Geometry check sheet. Reference: the model listing, model coordinates, mm. A direction names the side the tool comes from. Round coordinates to 2 decimals unless told otherwise and drop trailing zeros. Loops run counter-clockwise (first coordinate to the right, second up) from the corner with the lowest first, then second, coordinate; pieces in that order, holes last. Notation, with made-up numbers: (88, 36.25) - (130, 36.25) arc R24 cw to (130, 51.25) - close; hole circle Ø3 at (-32.5, 42). An arc over 180 degrees is marked (long way). Answer as CSV lines item,"result". Start each with the question number.
1) Thickness scan on line 1 along Y through (x, z) = (-45.25, 9.25); line 2 along X through (y, z) = (3.8, 14); line 3 along X through (y, z) = (0.25, 12.75). Record the ranges inside material, lowest first.
2) Access from +Z, -Z, +X, -X, +Y, -Y to the whole of each face (thin tool, end or side, straight path). Record for faces 1 (the flat face through (-49, 3, 13.787)), 2 (the flat face through (-48.043, 3, 8)), 3 (the flat face through (-50.143, 3, 8)), 4 (the cylindrical face through (-54.17, 1.49, 15.39)), 5 (the conical face through (-53.956, 0.191, 15.167)).
3) Cross-section at D-D on y = 1. Record the boundary of the cut face in (x, z), and give its area (3 significant figures).
4) Cross-section at C-C on z = 12. Record the boundary of the cut face in (x, y), and give its area (4 significant figures).
5) Depth check by flat-ended pin: P1, Ø1, axis at y = 3.5, z = 15, coming from the -X side; P2, Ø1.6, axis at y = 3, z = 8.5, coming from the +X side; P3, Ø1.6, axis at y = 4, z = 14.5, coming from the +X side. Enter the tip coordinate at first touch or a pass-through.
6) Cross-section at B-B on x = -52.75. Record the boundary of the cut face in (y, z).
7) Cross-section at A-A on y = 4. Record the boundary of the cut face in (x, z), and give its area (3 significant figures).
from build123d import *

# Parameters (mm, degrees)
EXTRUDE_1_DEPTH = 2.5
CHAMFER_1_SIZE  = 0.5
SKETCH_2_W      = 2.1
SKETCH_2_H      = 2
EXTRUDE_2_DEPTH = 2


with BuildPart() as part:
    # 草图1 → 凸台-拉伸1 (new body)
    with BuildSketch(Plane(origin=(0, 0, 0), x_dir=(1, 0, 0), z_dir=(0, 1, 0))):
        with BuildLine():
            Line((-53.192801429, -6.98717318), (-44.992801429, -6.98717318))
            ThreePointArc((-44.992801429, -6.98717318), (-44.002851935, -7.397223687), (-43.592801429, -8.38717318))
            Line((-43.592801429, -8.38717318), (-43.592801429, -14.38717318))
            ThreePointArc((-43.592801429, -14.38717318), (-44.002851935, -15.377122674), (-44.992801429, -15.78717318))
            Line((-44.992801429, -15.78717318), (-53.192801429, -15.78717318))
            ThreePointArc((-53.192801429, -15.78717318), (-54.182750923, -15.377122674), (-54.592801429, -14.38717318))
            Line((-54.592801429, -14.38717318), (-54.592801429, -8.38717318))
            ThreePointArc((-54.592801429, -8.38717318), (-54.182750923, -7.397223687), (-53.192801429, -6.98717318))
        make_face()
    extrude(amount=EXTRUDE_1_DEPTH)

    # 倒角1
    chamfer_1_edges = [part.edges().sort_by_distance(p)[0] for p in [
        (-49.092801429, 0, 6.98717318),
        (-44.002851935, 0, 7.397223687),
        (-43.592801429, 0, 11.38717318),
        (-44.002851935, 0, 15.377122674),
        (-49.092801429, 0, 15.78717318),
        (-54.182750923, 0, 15.377122674),
        (-54.592801429, 0, 11.38717318),
        (-54.182750923, 0, 7.397223687),
    ]]
    chamfer(chamfer_1_edges, length=CHAMFER_1_SIZE)

    # 草图2 → 凸台-拉伸2 (add)
    with BuildSketch(Plane(origin=(0, 2.5, 0), x_dir=(1, 0, 0), z_dir=(0, 1, 0))):
        with Locations((-49.092801429, -7.98717318)):
            Rectangle(SKETCH_2_W, SKETCH_2_H)
        with Locations((-49.092801429, -14.78717318)):
            Rectangle(SKETCH_2_W, SKETCH_2_H)
    extrude(amount=EXTRUDE_2_DEPTH)


solid = part.part
Answer block:
1,line 1,"y = 0 to 2.5"
1,line 2,"x = -50.14 to -48.04"
1,line 3,"x = -54.34 to -43.84"
2,face 1,"+X, -X, +Y"
2,face 2,"+Z, -Z, +X, +Y"
2,face 3,"+Z, -Z, -X, +Y"
2,face 4,"+Z, -X, +Y, -Y"
2,face 5,"+Z, -X, -Y"
3,outline,"(-54.59, 8.39) arc R1.4 ccw to (-53.19, 6.99) - (-44.99, 6.99) arc R1.4 ccw to (-43.59, 8.39) - (-43.59, 14.39) arc R1.4 ccw to (-44.99, 15.79) - (-53.19, 15.79) arc R1.4 ccw to (-54.59, 14.39) - close"
3,area,"95.1 mm^2"
4,outline,"(-54.59, 0.5) - (-54.09, 0) - (-44.09, 0) - (-43.59, 0.5) - (-43.59, 2.5) - (-54.59, 2.5) - close"
4,area,"27.25 mm^2"
5,P1,"stops at x = -50.14"
5,P2,"stops at x = -43.59"
5,P3,"stops at x = -48.04"
6,outline,"(0, 7.49) - (0.5, 6.99) - (2.5, 6.99) - (2.5, 15.79) - (0.5, 15.79) - (0, 15.29) - close"
7,outline,"(-50.14, 6.99) - (-48.04, 6.99) - (-48.04, 8.99) - (-50.14, 8.99) - close; (-50.14, 13.79) - (-48.04, 13.79) - (-48.04, 15.79) - (-50.14, 15.79) - close"
7,area,"8.40 mm^2"
